Design review of the part shown in the three views and the two pictorial views. Dimensions are in mm from the part's minimum x, y and z. Give positions to 0.01 mm unless a question says otherwise; leave off trailing zeros. Loops run counter-clockwise (first coordinate to the right, second up) from the corner with the lowest first, then second, coordinate; pieces in that order, holes last. Notation, with made-up numbers: (-16.75, 78) -> (-11.75, 78) arc R25 cw to (-11.75, 91) -> close; hole circle Ø8 at (14.25, -12). An arc over 180 degrees is marked (long way). Answer as CSV lines item,"result".
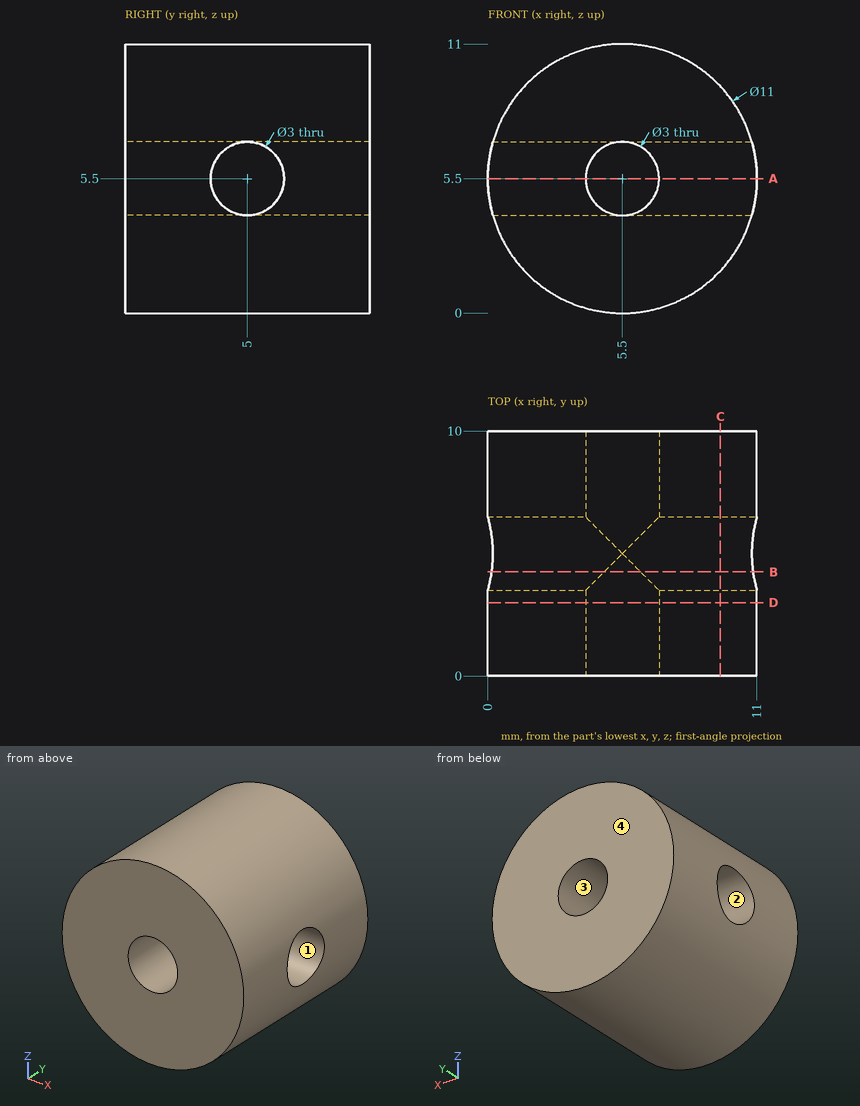
Q1. Clearance check with flat-ended pins moving along their axes: pin 1 Ø5 at (x, z) = (5.5, 5.5) entering from +Y; pin 2 Ø1.8 at (y, z) = (5, 5.5) entering from +X; pin 3 Ø1 at (y, z) = (6.5, 6.5) entering from +X; pin 4 Ø4 at (x, y) = (8.5, 8) entering from -Z. State where each tip first meets the part, or that it passes through.
Filled sheet:
pin 1,"stops at y = 10"
pin 2,"passes through"
pin 3,"stops at x = 10.98"
pin 4,"stops at z = 0.09"
Q2. We need section B-B, the plane y = 4.25. State the section outline as (x, z) points, and give its area (3 significant figures).
Filled sheet:
outline,"(0.16, 4.2) arc R5.5 ccw to (10.84, 4.2) -> (6.25, 4.2) arc R1.5 cw to (4.75, 4.2) -> close; (0.16, 6.8) -> (4.75, 6.8) arc R1.5 cw to (6.25, 6.8) -> (10.84, 6.8) arc R5.5 ccw to start"
area,"66.3 mm^2"
Q3. The part is to be moulded in two halves that separate along Y. For the marked faces 1, 2, 3 and 4, say which applies: pulls with the +Y half, pulls with the -Y half, needs draft (parallel to the pull), parting line crosses it, or undercut.
Filled sheet:
face 1,"undercut"
face 2,"undercut"
face 3,"needs draft"
face 4,"pulls with the +Y half"
Q4. We need section C-C, the plane x = 9.5. State the section outline as (y, z) points, and give its area (3 significant figures).
Filled sheet:
outline,"(0, 1.73) -> (10, 1.73) -> (10, 9.27) -> (0, 9.27) -> close; hole circle Ø3 at (5, 5.5)"
area,"68.4 mm^2"
Q5. To check wall thickness, follow probe 1 along Z at (x, y) = (5.5, 3.3); probe 2 along X at (y, z) = (8.75, 5.25); probe 3 along Z at (x, y) = (9.2, 5). State the ranges of each line that lie inside material, in increasing order. Write a range as from..to.
Filled sheet:
probe 1,"z = 0..4, 7..11"
probe 2,"x = 0.01..4.02, 6.98..10.99"
probe 3,"z = 1.43..4, 7..9.57"
Q6. We need section A-A, the plane z = 5.5. State the section outline as (x, y) points.
Filled sheet:
outline,"(0, 0) -> (4, 0) -> (4, 3.5) -> (0, 3.5) -> close; (0, 6.5) -> (4, 6.5) -> (4, 10) -> (0, 10) -> close; (7, 0) -> (11, 0) -> (11, 3.5) -> (7, 3.5) -> close; (7, 6.5) -> (11, 6.5) -> (11, 10) -> (7, 10) -> close"
Q7. We need section D-D, the plane y = 3. State the section outline as (x, z) points.
Filled sheet:
outline,"circle Ø11 at (5.5, 5.5); hole circle Ø3 at (5.5, 5.5)"
